Answer from the drawing. Dimensions are ordinates in mm from the lowest x, y and z of the part. A direction names the side the tool comes from. Coordinates: 2 decimals unless noted, no trailing zeros. Write each loop counter-clockwise with the first axis right and the second up, starting at its lowest first coordinate (ties: lowest second). Pieces come first, ordered by that corner, then holes.
1) Determine the mould class of the marked faces 4, 5 and 6 for opening direction X: +X half, -X half, draft (parallel to the pull), parting line (faces both ways), or undercut.
2) The part is cut by section B-B (x = 12.5). Determine the outline of the cut face in (y, z).
3) Each of these flat-tipped pins is pushed along its axis until it touches: pin 1 Ø10 at (x, y) = (7.5, 26.5) entering from -Z; pin 2 Ø1.4 at (x, z) = (13, 4) entering from -Y; pin 3 Ø3 at (x, z) = (8, 3) entering from -Y. Where does it stop, or does it pass through?
4) The part is cut by section C-C (z = 1.5). Determine the outline of the cut face in (x, y).
5) The part is cut by section A-A (y = 21.5). Determine the outline of the cut face in (x, z), then the cut area to 3 significant figures.
6) The part is cut by section D-D (x = 7). Determine the outline of the cut face in (y, z), then the cut area to 3 significant figures.
7) Which of the six approach directions +Z, -Z, +X, -X, +Y, -Y give full straight-line access (tool end or side, diameter ignored) to the marked faces 1, 2 and 3?
8) Find the intervals of material crossed by line 1 (X direction, y = 24, z = 3); line 2 (Y direction, x = 15, z = 5.25); line 3 (X direction, y = 22, z = 3.25), in increasing order.
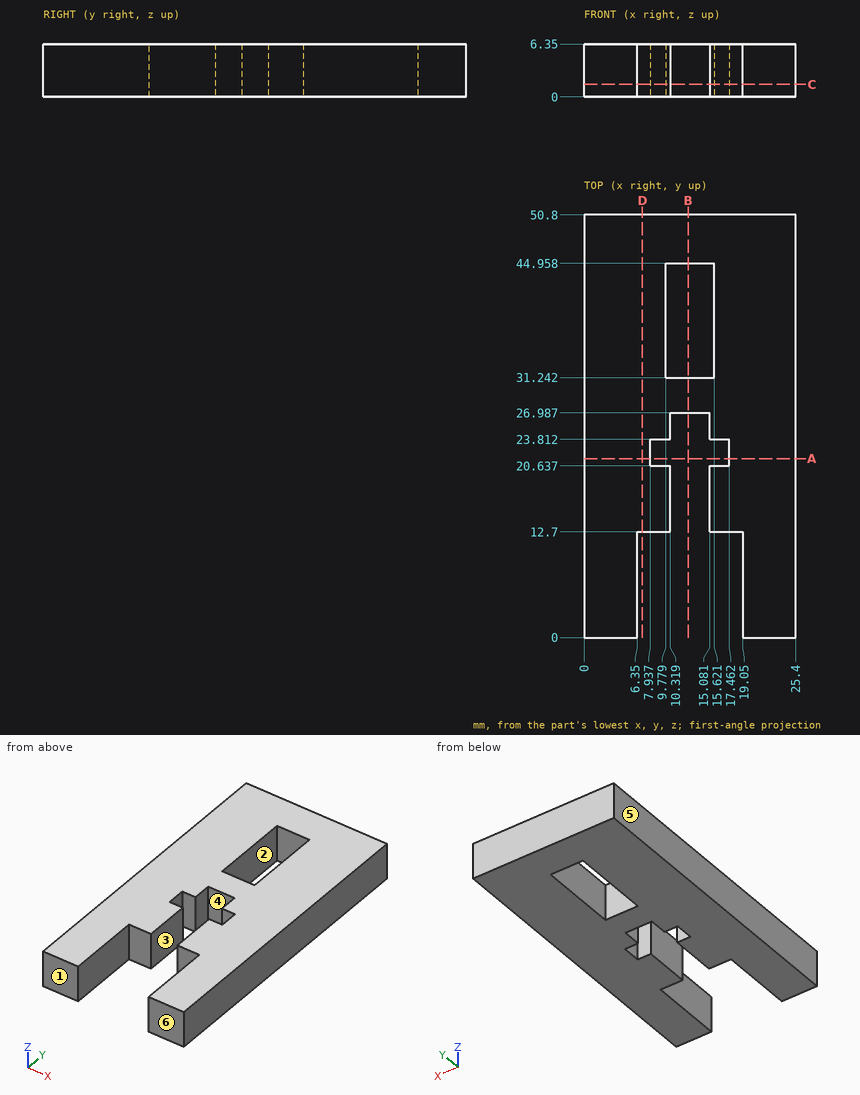
Reported:
1. face 4: undercut
1. face 5: -X half
1. face 6: draft
2. outline: (26.99, 0) - (31.24, 0) - (31.24, 6.35) - (26.99, 6.35) - close; (44.96, 0) - (50.8, 0) - (50.8, 6.35) - (44.96, 6.35) - close
3. pin 1: stops at z = 0
3. pin 2: stops at y = 26.99
3. pin 3: stops at y = 12.7
4. outline: (0, 0) - (6.35, 0) - (6.35, 12.7) - (10.32, 12.7) - (10.32, 20.64) - (7.94, 20.64) - (7.94, 23.81) - (10.32, 23.81) - (10.32, 26.99) - (15.08, 26.99) - (15.08, 23.81) - (17.46, 23.81) - (17.46, 20.64) - (15.08, 20.64) - (15.08, 12.7) - (19.05, 12.7) - (19.05, 0) - (25.4, 0) - (25.4, 50.8) - (0, 50.8) - close; hole (9.78, 31.24) - (15.62, 31.24) - (15.62, 44.96) - (9.78, 44.96) - close
5. outline: (0, 0) - (7.94, 0) - (7.94, 6.35) - (0, 6.35) - close; (17.46, 0) - (25.4, 0) - (25.4, 6.35) - (17.46, 6.35) - close
5. area: 101 mm2
6. outline: (12.7, 0) - (50.8, 0) - (50.8, 6.35) - (12.7, 6.35) - close
6. area: 242 mm2
7. face 1: +Z, -Z, +X, -X, -Y
7. face 2: +Z, -Z
7. face 3: +Z, -Z, -Y
8. line 1: x = 0 to 10.32, 15.08 to 25.4
8. line 2: y = 26.99 to 31.24, 44.96 to 50.8
8. line 3: x = 0 to 7.94, 17.46 to 25.4
